from build123d import *

# Parameters (mm, degrees)
F0_R     = 2.5
F0_R_2   = 2.875
F1_DEPTH = 3
F2_R     = 5
F3_R     = 10


with BuildPart() as f1:
    # F0 (on Top) → F1 (new body)
    with BuildSketch(Plane.XY):
        with BuildLine():
            Line((37.5, -12.5), (37.5, 12.5))
            Line((37.5, 12.5), (9.650635, 12.5))
            Line((9.650635, 12.5), (-12, 0))
            ThreePointArc((-12, 0), (-12.522727, -0.37363), (-13.107664, -0.63951))
            ThreePointArc((-13.107664, -0.63951), (-16.111338, -0.199497), (-17.5, 2.5))
            Line((-17.5, 2.5), (-17.5, 12.5))
            Line((-17.5, 12.5), (-37.5, 12.5))
            Line((-37.5, 12.5), (-37.5, 5.5))
            Line((-37.5, 5.5), (-41.5, 5.5))
            ThreePointArc((-41.5, 5.5), (-47, 0), (-41.5, -5.5))
            Line((-41.5, -5.5), (-37.5, -5.5))
            Line((-37.5, -5.5), (-37.5, -12.5))
            Line((-37.5, -12.5), (-9.650635, -12.5))
            Line((-9.650635, -12.5), (12.679396, 0.392249))
            ThreePointArc((12.679396, 0.392249), (15.908496, 0.310842), (17.5, -2.5))
            Line((17.5, -2.5), (17.5, -12.5))
            Line((17.5, -12.5), (37.5, -12.5))
        make_face()
        with Locations((-41.5, 0)):
            Circle(F0_R, mode=Mode.SUBTRACT)
        with Locations((-30.5, 0)):
            Circle(F0_R_2, mode=Mode.SUBTRACT)
        with Locations((30.5, 0)):
            Circle(F0_R_2, mode=Mode.SUBTRACT)
        with BuildLine():
            ThreePointArc((-13.107664, -0.63951), (-12.522727, -0.37363), (-12, 0))
            Line((-12, 0), (-13.107664, -0.63951))
        make_face()
    extrude(amount=F1_DEPTH)

    # F2
    f2_edges = [f1.edges().sort_by_distance(p)[0] for p in [
        (-17.5, 12.5, 1.5),
        (17.5, -12.5, 1.5),
        (37.5, -12.5, 1.5),
        (37.5, 12.5, 1.5),
        (-37.5, -12.5, 1.5),
        (-37.5, 12.5, 1.5),
    ]]
    fillet(f2_edges, radius=F2_R)

    # F3
    f3_edges = [f1.edges().sort_by_distance(p)[0] for p in [
        (-9.650635, -12.5, 1.5),
        (9.650635, 12.5, 1.5),
    ]]
    fillet(f3_edges, radius=F3_R)


solid = f1.part
Geometry: final body of the model. Coordinates: model frame, mm. A direction names the side the tool comes from. Round coordinates to 2 decimals unless told otherwise and drop trailing zeros. Loops run counter-clockwise (first coordinate to the right, second up) from the corner with the lowest first, then second, coordinate; pieces in that order, holes last.
Q1. Pin query (flat end, axial travel): P1, Ø4.5, axis at x = 30.5, y = 0, coming from the -Z side; P2, Ø6, axis at x = -41.5, y = 0, coming from the -Z side; P3, Ø1, axis at x = 20.5, z = 1.5, coming from the -Y side; P4, Ø1.5, axis at x = -39, z = 2, coming from the +Y side. Return the tip coordinate at first contact, or that it passes through.
Q2. Material intervals for L1, parallel to Y at x = -41.5, z = 1.25; L2, parallel to Y at x = 30.5, z = 0.95 (3 decimals); L3, parallel to X at y = -0.5, z = 2.8, sorted ascending.
Q3. Access query for faces 1 (the cylindrical face through (-9.71, -12.15, 1.52)), 2 (the flat face through (-37.5, 7, 1)), 3 (the cylindrical face through (36.07, -11, 1.52)), 4 (the cylindrical face through (-18.93, 11, 1.52)). Directions: +Z, -Z, +X, -X, +Y, -Y. A direction counts if a zero-diameter tool reaches every point of the face in a straight line with its end or side. Return the directions, or none.
Q4. Section D-D on y = 1.75. Return loops of the section in (x, z).
Q5. Section A-A on z = 1.3. State how many separate pieces and enclosed holes the cut face has, plus the area to 3 significant figures.
Q6. Pull-direction query (X, two-part tool) for faces 5 (the cylindrical face through (36.07, 11, 1.52)), 6 (the flat face through (23, 12.5, 1)), 7 (the cylindrical face through (15.868, 0.335, 1.479)); classes: released by +X, released by -X, zero draft, split by the parting line, or undercut.
Q7. Section B-B on y = 10. Return loops of the section in (x, z), plus the area to 3 significant figures.
Q8. Section C-C on x = 30.5. Return loops of the section in (y, z) (3 decimals), plus the area to 4 significant figures.
Evaluation:
1. P1: passes through
1. P2: stops at z = 0
1. P3: stops at y = -12.27
1. P4: stops at y = 5.5
2. L1: y = -5.5 to -2.5, 2.5 to 5.5
2. L2: y = -12.5 to -2.875, 2.875 to 12.5
2. L3: x = -46.98 to -43.95, -39.05 to -33.33, -27.67 to -15.6, -12.87 to 11.13, 16.82 to 27.67, 33.33 to 37.5
3. face 1: +Z, -Z, -Y
3. face 2: +Z, -Z, -X, +Y
3. face 3: +Z, -Z, +X, -Y
3. face 4: +Z, -Z, +Y
4. outline: (-46.71, 0) - (-43.29, 0) - (-43.29, 3) - (-46.71, 3) - close; (-39.71, 0) - (-32.78, 0) - (-32.78, 3) - (-39.71, 3) - close; (-28.22, 0) - (-17.41, 0) - (-17.41, 3) - (-28.22, 3) - close; (-8.97, 0) - (28.22, 0) - (28.22, 3) - (-8.97, 3) - close; (32.78, 0) - (37.5, 0) - (37.5, 3) - (32.78, 3) - close
5. separate pieces: 1
5. enclosed holes: 3
5. area: 1,450 mm2
6. face 5: released by +X
6. face 6: zero draft
6. face 7: undercut
7. outline: (-36.83, 0) - (-18.17, 0) - (-18.17, 3) - (-36.83, 3) - close; (5.32, 0) - (36.83, 0) - (36.83, 3) - (5.32, 3) - close
7. area: 151 mm2
8. outline: (-12.5, 0) - (-2.875, 0) - (-2.875, 3) - (-12.5, 3) - close; (2.875, 0) - (12.5, 0) - (12.5, 3) - (2.875, 3) - close
8. area: 57.75 mm2
